```python
from build123d import *

# Parameters (mm, degrees)
F1_DEPTH = 25.4
F2_R     = 2.5399
F3_R     = 2.54


# Not quite as in the source:
# - a fillet or chamfer is up to 0.001 mm smaller than in the source, because OpenCascade refuses the exact size


with BuildPart() as f1:
    # F0 (on Front) → F1 (new body)
    with BuildSketch(Plane.XZ):
        with BuildLine():
            ThreePointArc((-13.5573409498, -17.4706149846), (0, -13.5498725689), (13.5573409498, -17.4706149846))
            Line((13.5573409498, -17.4706149846), (13.5573409498, 36.2410636034))
            ThreePointArc((13.5573409498, 36.2410636034), (0, 32.3203211877), (-13.5573409498, 36.2410636034))
            Line((-13.5573409498, 36.2410636034), (-13.5573409498, -17.4706149846))
        make_face()
        with BuildLine():
            ThreePointArc((-13.5573409498, 36.2410636034), (0, 32.3203211877), (13.5573409498, 36.2410636034))
            ThreePointArc((13.5573409498, 36.2410636034), (22.2431614224, 45.4564812533), (25.4, 57.7203211877))
            ThreePointArc((25.4, 57.7203211877), (21.419954319, 71.3711657393), (10.7271214983, 80.7439799838))
            Line((10.7271214983, 80.7439799838), (17.3568471858, 60.3397823797))
            Line((17.3568471858, 60.3397823797), (0, 47.7292947471))
            Line((0, 47.7292947471), (-17.3568471858, 60.3397823797))
            Line((-17.3568471858, 60.3397823797), (-10.7271214983, 80.7439799838))
            ThreePointArc((-10.7271214983, 80.7439799838), (-25.34879032, 59.3324096814), (-13.5573409498, 36.2410636034))
        make_face()
        with BuildLine():
            ThreePointArc((9.2408497758, -62.6092617289), (20.9747179278, -53.2754164625), (25.4, -38.9498725689))
            ThreePointArc((25.4, -38.9498725689), (22.2431614224, -26.6860326345), (13.5573409498, -17.4706149846))
            ThreePointArc((13.5573409498, -17.4706149846), (0, -13.5498725689), (-13.5573409498, -17.4706149846))
            ThreePointArc((-13.5573409498, -17.4706149846), (-25.2846540922, -41.3677781576), (-9.2408497758, -62.6092617289))
            Line((-9.2408497758, -62.6092617289), (-18.3499921745, -46.8317642808))
            Line((-18.3499921745, -46.8317642808), (-9.1749960873, -30.9402048984))
            Line((-9.1749960873, -30.9402048984), (9.1749960873, -30.9402048984))
            Line((9.1749960873, -30.9402048984), (18.3499921745, -46.8317642808))
            Line((18.3499921745, -46.8317642808), (9.2408497758, -62.6092617289))
        make_face()
    extrude(amount=F1_DEPTH)

    # F2 (radius 2.54 in the source; OpenCascade refuses exactly that, so slightly less here)
    f2_edges = [f1.edges().sort_by_distance(p)[0] for p in [
        (-13.762494, -25.4, -38.885985),
        (0, -25.4, -30.940205),
        (13.762494, -25.4, -38.885985),
        (-13.795421, -25.4, -54.720513),
        (13.795421, -25.4, -54.720513),
        (25.284654, -25.4, -41.367778),
        (-25.284654, -25.4, -41.367778),
        (-13.557341, -25.4, 9.385224),
        (-25.34879, -25.4, 59.33241),
        (-8.678424, -25.4, 54.034539),
        (-14.041984, -25.4, 70.541881),
        (14.041984, -25.4, 70.541881),
        (8.678424, -25.4, 54.034539),
        (25.34879, -25.4, 59.33241),
        (13.557341, -25.4, 9.385224),
    ]]
    fillet(f2_edges, radius=F2_R)

    # F3
    f3_edges = [f1.edges().sort_by_distance(p)[0] for p in [
        (25.34879, 0, 59.33241),
        (14.041984, 0, 70.541881),
        (8.678424, 0, 54.034539),
        (-14.041984, 0, 70.541881),
        (-8.678424, 0, 54.034539),
        (-25.34879, 0, 59.33241),
        (13.557341, 0, 9.385224),
        (-13.557341, 0, 9.385224),
        (25.284654, 0, -41.367778),
        (13.762494, 0, -38.885985),
        (13.795421, 0, -54.720513),
        (0, 0, -30.940205),
        (-13.762494, 0, -38.885985),
        (-25.284654, 0, -41.367778),
        (-13.795421, 0, -54.720513),
    ]]
    fillet(f3_edges, radius=F3_R)


solid = f1.part
```
Verification items for the finished model (mm, model axes). A direction names the side the tool comes from. Coordinates: 2 decimals unless noted, no trailing zeros. Write each loop counter-clockwise with the first axis right and the second up, starting at its lowest first coordinate (ties: lowest second). Pieces come first, ordered by that corner, then holes. Notation, with made-up numbers: M 81,-25 L 140,-25 A17 cw 140,-20 Z; hole C -27,36.5 d8. An arc over 180 degrees is marked long. Answer as a JSON object with one key per item and string values. Group by question number.
(1) Tool access check on faces 4 (the face through (12.83, -0.76, 9.78)), 5 (the face through (-14.09, -12.56, 70.4)), 6 (the face through (-9.27, -0.724, 53.52)), 7 (the face through (-13.557, -13, 10)), 8 (the face through (8.962, -24.636, 53.345)). Record the directions out of +Z, -Z, +X, -X, +Y, -Y that give a thin tool (end or side, any length) a straight path to the whole face; none if there is none.
(2) Gauge pin test, flat ends, axial feed: pin 1 (10 mm diameter, centred on x = 5, y = -17.5, fed in from +Z); pin 2 (6 mm diameter, centred on x = 1.5, y = -13, fed in from +Z); pin 3 (10 mm diameter, centred on y = -8, z = 28.5, fed in from +X). Record the tip position at first contact, or that the pin passes through.
(3) Cross-section at B-B, the plane y = -8.75. Record the cut outline in (x, z) (3 decimals).
(4) Material ranges on line 1 (Y direction, x = -23, z = 54.5); line 2 (X direction, y = -10, z = 4.5); line 3 (Z direction, x = -10, y = -12.25), recorded low to high.
(5) Release check for a two-part mould opening along Z. For faces 1 (the face through (0, 0, 11)), 2 (the face through (13.557, -13, 9)), 3 (the face through (0, -13, -30.94)) record: +Z half, -Z half, draft (parallel to the pull), parting line (faces both ways), or undercut.
(6) Cross-section at A-A, the plane z = 8. Record the cut outline in (x, y).
Reply:
{
 "1": {"face 4": "+X, +Y", "face 5": "+Y, -Y", "face 6": "+Y", "face 7": "-X, +Y, -Y", "face 8": "-Y"},
 "2": {"pin 1": "z = 54.99", "pin 2": "z = 51", "pin 3": "x = 13.56"},
 "3": {"outline": "M -18.35,-46.832 L -9.175,-30.94 L 9.175,-30.94 L 18.35,-46.832 L 9.241,-62.609 A25.4 ccw 13.557,-17.471 L 13.557,36.241 A25.4 ccw 10.727,80.744 L 17.357,60.34 L 0,47.729 L -17.357,60.34 L -10.727,80.744 A25.4 ccw -13.557,36.241 L -13.557,-17.471 A25.4 ccw -9.241,-62.609 Z"},
 "4": {"line 1": "-25.37 to -0.03", "line 2": "-13.56 to 13.56", "line 3": "-62.3 to -61.29, -32.37 to 54.99"},
 "5": {"face 1": "draft", "face 2": "undercut", "face 3": "-Z half"},
 "6": {"outline": "M -13.56,-22.86 A2.54 ccw -11.02,-25.4 L 11.02,-25.4 A2.54 ccw 13.56,-22.86 L 13.56,-2.54 A2.54 ccw 11.02,0 L -11.02,0 A2.54 ccw -13.56,-2.54 Z"}
}
